from build123d import *

# Parameters (mm, degrees)
SKETCH1_R                     = 12.5
MIL_CONFIGURED_CAP_25_1_DEPTH = 58.05
IZIM3_W                       = 30
IZIM3_H                       = 2.5
IZIM3_W_2                     = 6.95
PAH1_SIZE                     = 0.5
PAH2_SIZE                     = 1.5
IZIM6_W                       = 3
IZIM6_H                       = 1.5
PAH3_SIZE                     = 0.5


with BuildPart() as part:
    # Sketch1 → Mil - configured CAP=25(1) (new body)
    with BuildSketch(Plane.YX.offset(-29.025)):
        Circle(SKETCH1_R)
    extrude(amount=MIL_CONFIGURED_CAP_25_1_DEPTH)

    # Çizim3 → Kes-Döndür1 (revolve, cut)
    with BuildSketch(Plane(origin=(0, 0, 0), x_dir=(0, 0, -1), z_dir=(1, 0, 0)), mode=Mode.PRIVATE) as kes_d_nd_r1_sk:
        with Locations((14.025, 11.25)):
            Rectangle(IZIM3_W, IZIM3_H)
        with Locations((-25.55, 11.25)):
            Rectangle(IZIM3_W_2, IZIM3_H)
    revolve(kes_d_nd_r1_sk.sketch.rotate(Axis((0, 0, -29.025), (0, 0, -1)), 90), axis=Axis((0, 0, -29.025), (0, 0, -1)), mode=Mode.SUBTRACT)

    # Çizim4 → M8 Dişli Delik1 (revolve, cut)
    with BuildSketch(Plane(origin=(0, 0, 29.025), x_dir=(0, -1, 0), z_dir=(1, 0, 0))):
        Polygon((0, 0), (0, 24.292926105), (3.4, 22.25), (3.4, 0), align=None)
    m8_di_li_delik1 = revolve(axis=Axis((0, 0, 35.375), (0, 0, -1)), mode=Mode.SUBTRACT)

    # Aynalama1: M8 Dişli Delik1 across plane
    add(m8_di_li_delik1.mirror(Plane.XY), mode=Mode.SUBTRACT)

    # Pah1
    pah1_edges = [part.edges().sort_by_distance(p)[0] for p in [
        (-10, 0, 29.025),
        (0, 3.4, 29.025),
        (0, 3.4, -29.025),
        (-10, 0, -29.025),
        (0, -12.5, 0.975),
    ]]
    chamfer(pah1_edges, length=PAH1_SIZE)

    # Pah2
    pah2_edges = [part.edges().sort_by_distance(p)[0] for p in [
        (0, -12.5, 22.075),
    ]]
    chamfer(pah2_edges, length=PAH2_SIZE)

    # Çizim6 → Kes-Döndür2 (revolve, cut)
    with BuildSketch(Plane(origin=(0, 0, 0), x_dir=(0, 0, -1), z_dir=(1, 0, 0)), mode=Mode.PRIVATE) as kes_d_nd_r2_sk:
        with Locations((-20.575, 11.75)):
            Rectangle(IZIM6_W, IZIM6_H)
    revolve(kes_d_nd_r2_sk.sketch.rotate(Axis((0, 0, 29.025), (0, 0, 1)), 180), axis=Axis((0, 0, 29.025), (0, 0, 1)), mode=Mode.SUBTRACT)

    # Pah3
    pah3_edges = [part.edges().sort_by_distance(p)[0] for p in [
        (0, -12.5, 19.075),
    ]]
    chamfer(pah3_edges, length=PAH3_SIZE)


solid = part.part
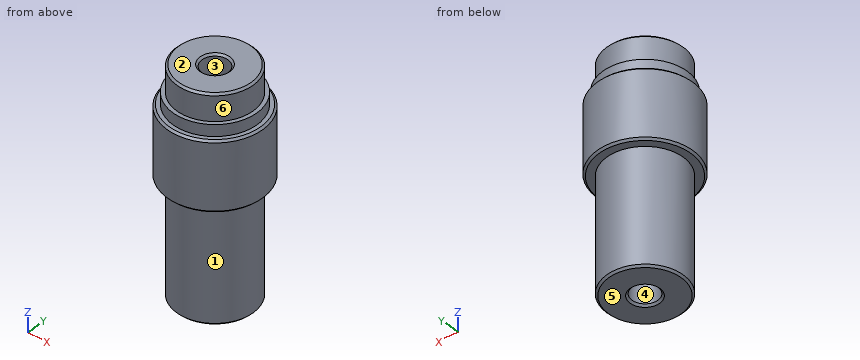
Here's how the part is built. I have some questions about the finished solid (model axes, mm). Face numbers are marked on the shaded views. A direction names the side the tool comes from. Coordinates: 2 decimals unless noted, no trailing zeros. Write each loop counter-clockwise with the first axis right and the second up, starting at its lowest first coordinate (ties: lowest second). Pieces come first, ordered by that corner, then holes. Notation, with made-up numbers: (48.5, -18) - (92.5, -18) arc R23 cw to (92.5, 15) - close; hole circle Ø10 at (-1, 58.5). An arc over 180 degrees is marked (long way). Use one line per item in the form item = value.
1) I need wall thicknesses on line 1 (Y direction, x = 0, z = 23.5); line 2 (X direction, y = 0, z = 12); line 3 (Z direction, x = -6.5, y = 9.75) (3 decimals). Which ranges of each line are inside material? Lowest first, please.
Solved:
line_1 = -10 to -3.4, 3.4 to 10
line_2 = -12.5 to -3.4, 3.4 to 12.5
line_3 = 0.975 to 19.075
2) On a 3-axis mill with a long thin cutter (end or side, diameter ignored), from which of +Z, -Z, +X, -X, +Y, -Y can I reach the whole of each face in a straight line? I mean the marked faces 5 and 6. Say none if no direction works.
Solved:
face_5 = -Z, +X, -X, +Y, -Y
face_6 = +Z
3) Thinking about a two-plate mould opening in X: for the marked faces 1, 2, 3 and 4, which applies, released by +X, released by -X, zero draft, split by the parting line, or undercut?
Solved:
face_1 = split by the parting line
face_2 = zero draft
face_3 = undercut
face_4 = undercut
4) I'm going to push flat-ended pins straight in: P1, Ø1.5, axis at x = 3, z = -4.5, coming from the -Y side; P2, Ø5, axis at x = 3, z = 16.5, coming from the +Y side; P3, Ø4, axis at y = -10, z = 0.5, coming from the -X side. Where does each tip first touch, or does it pass through?
Solved:
P1 = -9.74
P2 = 12.49
P3 = -9.39
5) Suppose I cut it at A-A, the plane z = 15. Write out the boundary of the cut face in (x, y).
Solved:
outline = circle Ø25 at (0, 0); hole circle Ø6.8 at (0, 0)
